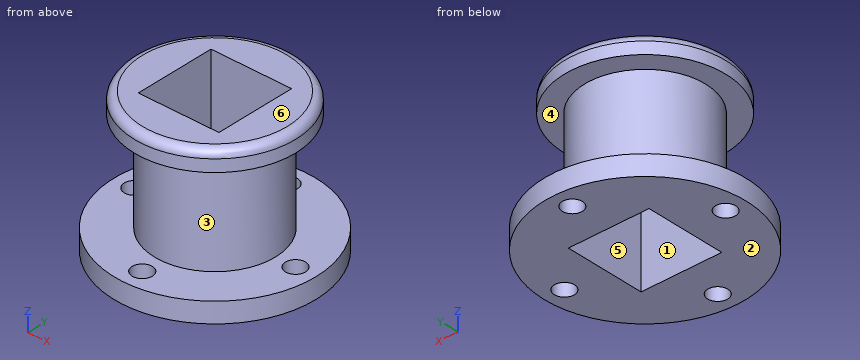
```python
from build123d import *

# Parameters (mm, degrees)
F0_R      = 38.1
F1_DEPTH  = 63.5
F2_R      = 63.5
F3_DEPTH  = 12.7
F4_R      = 6.35
F5_DEPTH  = 25.4
F6_R      = 50.8
F7_DEPTH  = 12.7
F8_R      = 5.08
F9_W      = 50.8
F9_H      = 50.8
F10_DEPTH = 132.842


with BuildPart() as f1:
    # F0 (on Top) → F1 (new body)
    with BuildSketch(Plane.XY):
        Circle(F0_R)
    extrude(amount=F1_DEPTH)

    # F2 (on Top) → F3 (join)
    with BuildSketch(Plane.XY):
        Circle(F2_R)
    extrude(amount=-F3_DEPTH)

    # F4 (on face) → F5 (cut)
    with BuildSketch(Plane.XY):
        with Locations((-50.8, 0)):
            Circle(F4_R)
        with Locations((0, 50.8)):
            Circle(F4_R)
        with Locations((50.8, 0)):
            Circle(F4_R)
        with Locations((0, -50.8)):
            Circle(F4_R)
    extrude(amount=-F5_DEPTH, mode=Mode.SUBTRACT)

    # F6 (on face) → F7 (join)
    with BuildSketch(Plane.XY.offset(63.5)):
        Circle(F6_R)
    extrude(amount=F7_DEPTH)

    # F8
    f8_edges = [f1.edges().sort_by_distance(p)[0] for p in [
        (-50.8, 0, 76.2),
    ]]
    fillet(f8_edges, radius=F8_R)

    # F9 (on face) → F10 (cut)
    with BuildSketch(Plane.XY.offset(76.2)):
        Rectangle(F9_W, F9_H)
    extrude(amount=-F10_DEPTH, mode=Mode.SUBTRACT)


solid = f1.part
```
Source: CAD feature listing. Evaluate the final solid. Frame: model axes, mm. Face numbers are marked on the shaded views. A direction names the side the tool comes from. Round coordinates to 2 decimals unless told otherwise and drop trailing zeros. Loops run counter-clockwise (first coordinate to the right, second up) from the corner with the lowest first, then second, coordinate; pieces in that order, holes last.
1. Section query D-D on z = 13.5. Output: boundary loops of the cut face in (x, y).
2. Section query C-C on x = 53. Output: boundary loops of the cut face in (y, z) (3 decimals), and give its area (3 significant figures).
3. Mould query, pull axis Y, two halves, no side actions, for the marked faces 1, 2 and 3. Classes: released by +Y, released by -Y, zero draft, split by the parting line, or undercut.
4. Ray query, L1, parallel to Y at x = 0, z = -4; L2, parallel to Z at x = -43, y = -13; L3, parallel to X at y = 44, z = 70. Return the intervals inside material, ascending.
5. Access query for the marked faces 4, 5 and 6. Directions: +Z, -Z, +X, -X, +Y, -Y. A direction counts if a zero-diameter tool reaches every point of the face in a straight line with its end or side. Return the directions, or none.
6. Section query A-A on y = 0. Output: boundary loops of the cut face in (x, z).
7. Contact query for flat-ended pins moving along their axis: pin 1 (15 mm diameter, centred on x = -4, z = 51.5, fed in from -Y); pin 2 (15 mm diameter, centred on y = -11.5, z = 35.5, fed in from -X); pin 3 (1 mm diameter, centred on y = -10, z = 7.5, fed in from -X); pin 4 (1.5 mm diameter, centred on y = -39, z = 37, fed in from +X). Output: stop coordinate, or through.
Answers below:
1. outline: circle Ø76.2 at (0, 0); hole (-25.4, -25.4) - (25.4, -25.4) - (25.4, 25.4) - (-25.4, 25.4) - close
2. outline: (-34.975, -12.7) - (-5.957, -12.7) - (-5.957, 0) - (-34.975, 0) - close; (5.957, -12.7) - (34.975, -12.7) - (34.975, 0) - (5.957, 0) - close
2. area: 737 mm2
3. face 1: undercut
3. face 2: zero draft
3. face 3: split by the parting line
4. L1: y = -63.5 to -57.15, -44.45 to -25.4, 25.4 to 44.45, 57.15 to 63.5
4. L2: z = -12.7 to 0, 63.5 to 76.2
4. L3: x = -25.39 to 25.39
5. face 4: none
5. face 5: +Z, -Z
5. face 6: +Z, +X, -X, +Y, -Y
6. outline: (-63.5, -12.7) - (-57.15, -12.7) - (-57.15, 0) - (-63.5, 0) - close; (-50.8, 63.5) - (-38.1, 63.5) - (-38.1, 0) - (-44.45, 0) - (-44.45, -12.7) - (-25.4, -12.7) - (-25.4, 76.2) - (-45.72, 76.2) arc R5.08 ccw to (-50.8, 71.12) - close; (25.4, -12.7) - (44.45, -12.7) - (44.45, 0) - (38.1, 0) - (38.1, 63.5) - (50.8, 63.5) - (50.8, 71.12) arc R5.08 ccw to (45.72, 76.2) - (25.4, 76.2) - close; (57.15, -12.7) - (63.5, -12.7) - (63.5, 0) - (57.15, 0) - close
7. pin 1: stops at y = -38.1
7. pin 2: stops at x = -37.89
7. pin 3: stops at x = -36.9
7. pin 4: passes through
